Design review of the part built by this model. Coordinates are the model's own, in mm. Face numbers are marked on the shaded views. Give positions to 0.01 mm unless a question says otherwise; leave off trailing zeros. Order: outer loops, then holes, each group sorted by start corner. A loop starts at its lowest first (then second) coordinate and runs counter-clockwise, first axis right, second up. Notation, with made-up numbers: (17.5, -34) -> (76.5, -34) arc R26 cw to (76.5, -5) -> close; hole circle Ø9 at (-32, -10.5). An arc over 180 degrees is marked (long way). Use a Markdown table: item, result. Add a question column.
```python
from build123d import *

# Parameters (mm, degrees)
F1_DEPTH = 12.5
F2_R     = 0.2
F3_R     = 0.2


with BuildPart() as f1:
    # F0 (on Front) → F1 (new body)
    with BuildSketch(Plane.XZ):
        with BuildLine():
            Line((28.5, 4), (7, 4))
            Line((7, 4), (7, 3.5))
            Line((7, 3.5), (0, 3.5))
            Line((0, 3.5), (-7, 3.5))
            Line((-7, 3.5), (-7, 4))
            Line((-7, 4), (-28.5, 4))
            Line((-28.5, 4), (-28.5, 0))
            Line((-28.5, 0), (-28.5, -0.572795))
            ThreePointArc((-28.5, -0.572795), (-0.117692, -4.001252), (28.189545, 0))
            ThreePointArc((28.189545, 0), (28.344804, 0.043215), (28.5, 0.086657))
            Line((28.5, 0.086657), (28.5, 4))
        make_face()
    extrude(amount=F1_DEPTH)

    # F2
    f2_edges = [f1.edges().sort_by_distance(p)[0] for p in [
        (-7, -6.25, 3.5),
    ]]
    fillet(f2_edges, radius=F2_R)

    # F3
    f3_edges = [f1.edges().sort_by_distance(p)[0] for p in [
        (7, -6.25, 3.5),
    ]]
    fillet(f3_edges, radius=F3_R)


solid = f1.part
```
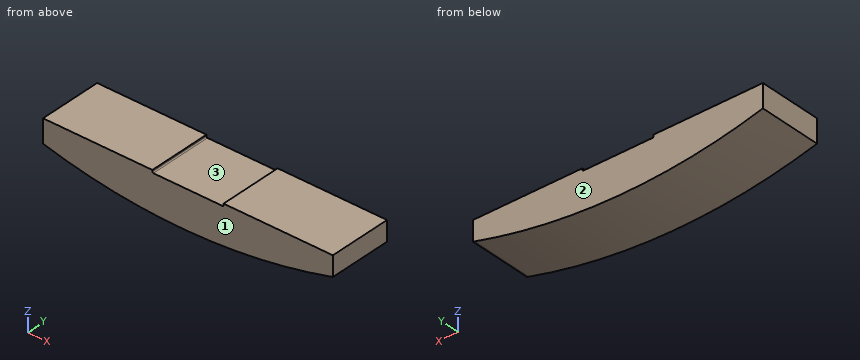
1) Add section A-A (y = -7). Give the boundary of the cut face in (x, z).
2) Add section C-C (x = -19.5). Give the boundary of the cut face in (y, z), then the cut area to 3 significant figures.
3) The part is to be moulded in two halves that separate along Y. For the marked faces 1, 2 and 3, say which applies: +Y half, -Y half, draft (parallel to the pull), parting line (faces both ways), or undercut.
4) Add section B-B (z = -1.25). Give the boundary of the cut face in (x, y).
5) For L1, parallel to Z at x = -2, y = -3.75; L2, parallel to Z at x = 24.5, y = -3.75, list the stretches that pass through material, from the lowest coordinate up. Write a range as [from, to].
6) Insertion check: pin 1 (5 mm diameter, centred on x = 9, y = -8.5, fed in from -Z) (3 decimals). The pin has a flat end and moves straight along its axis. Give the tip position at first contact, or say it passes through.
Worked answers:
| question | item | result |
|---|---|---|
| 1 | outline | (-28.5, -0.57) arc R110 ccw to (28.19, 0) arc R110.25 ccw to (28.5, 0.09) -> (28.5, 4) -> (7, 4) -> (7, 3.7) arc R0.2 cw to (6.8, 3.5) -> (-6.8, 3.5) arc R0.2 cw to (-7, 3.7) -> (-7, 4) -> (-28.5, 4) -> close |
| 2 | outline | (-12.5, -2.48) -> (0, -2.48) -> (0, 4) -> (-12.5, 4) -> close |
| 2 | area | 81.0 mm^2 |
| 3 | face 1 | -Y half |
| 3 | face 2 | +Y half |
| 3 | face 3 | draft |
| 4 | outline | (-25.7, -12.5) -> (23.24, -12.5) -> (23.24, 0) -> (-25.7, 0) -> close |
| 5 | L1 | [-4, 3.5] |
| 5 | L2 | [-0.96, 4] |
| 6 | pin 1 | z = -3.735 |
